Here's how the part is built. I have some questions about the finished solid (model axes, mm). Face numbers are marked on the shaded views. A direction names the side the tool comes from. Round coordinates to 2 decimals unless told otherwise and drop trailing zeros. Order: outer loops, then holes, each group sorted by start corner. A loop starts at its lowest first (then second) coordinate and runs counter-clockwise, first axis right, second up. Notation, with made-up numbers: M 14,-5.75 L 33,-5.75 A12 ccw 33,9.25 Z; hole C -38,82 d3. An arc over 180 degrees is marked long. Use one line per item in the form item = value. Start each with the question number.
```python
from build123d import *

# Parameters (mm, degrees)
SKETCH1_R           = 1.5
SKETCH1_W           = 3
SKETCH1_H           = 3
BOSS_EXTRUDE1_DEPTH = 3
FILLET1_R           = 4


with BuildPart() as part:
    # Sketch1 → Boss-Extrude1 (new body)
    # profile 1 of 3: a face of its own
    with BuildSketch(Plane(origin=(0, 0, 0), x_dir=(1, 0, 0), z_dir=(0, 1, 0))):
        Polygon((14.5, 10), (-1.5, 10), (-1.5, 0), (-8.5, 0), (-11.5, 0), (-14.5, 0), (-14.5, -10), (-11.5, -10), (-8.5, -10), (14.5, -10), align=None)
        with Locations(Location((6.5, 5.75, 0), (0, 0, 270))):
            Circle(SKETCH1_R, mode=Mode.SUBTRACT)
    # profile 2 of 3: a face of its own
    with BuildSketch(Plane(origin=(0, 0, 0), x_dir=(1, 0, 0), z_dir=(0, 1, 0))):
        with Locations((-10, -11.5)):
            Rectangle(SKETCH1_W, SKETCH1_H)
    # profile 3 of 3: a face of its own
    with BuildSketch(Plane(origin=(0, 0, 0), x_dir=(1, 0, 0), z_dir=(0, 1, 0))):
        with Locations((-10, 1.5)):
            Rectangle(SKETCH1_W, SKETCH1_H)
    extrude(amount=BOSS_EXTRUDE1_DEPTH)

    # Fillet1
    # the kernel refuses this fillet: 4 mm, written as the material it adds along each edge
    with BuildSketch(Plane(origin=(-8.5, 0, 0), x_dir=(1, 0, 0), z_dir=(0, 1, 0))) as fillet1_piece_1:
        with BuildLine():
            CenterArc((3.872983346, 4), FILLET1_R, 194.477512186, 75.522487814)
            Line((0, 3), (0, 0))
            Line((0, 0), (3.872983346, 0))
        make_face()
    extrude(amount=3)
    with BuildSketch(Plane(origin=(-8.5, 0, 10), x_dir=(1, 0, 0), z_dir=(0, 1, 0))) as fillet1_piece_2:
        with BuildLine():
            CenterArc((3.872983346, -4), FILLET1_R, 90, 75.522487814)
            Line((0, -3), (0, 0))
            Line((0, 0), (3.872983346, 0))
        make_face()
    extrude(amount=3)
    with BuildSketch(Plane(origin=(-1.5, 0, 0), x_dir=(0, 0, -1), z_dir=(0, 1, 0))) as fillet1_piece_3:
        with BuildLine():
            CenterArc((FILLET1_R, FILLET1_R), FILLET1_R, 180, 90)
            Line((0, FILLET1_R), (0, 0))
            Line((0, 0), (FILLET1_R, 0))
        make_face()
    extrude(amount=3)
    # the kernel refuses this fillet: 4 mm, written as the material it takes off along each edge
    with BuildSketch(Plane(origin=(14.5, -10, 10), x_dir=(0, 0, -1), z_dir=(0, 1, 0)), Plane(origin=(14.5, -10, -10), x_dir=(-1, 0, 0), z_dir=(0, 1, 0))) as fillet1_2_piece_1:
        with BuildLine():
            CenterArc((FILLET1_R, FILLET1_R), FILLET1_R, 180, 90)
            Line((0, FILLET1_R), (0, 0))
            Line((0, 0), (FILLET1_R, 0))
        make_face()
    extrude(amount=23, mode=Mode.SUBTRACT)
    with BuildSketch(Plane(origin=(-1.5, -10, -10), x_dir=(1, 0, 0), z_dir=(0, 1, 0))) as fillet1_2_piece_2:
        with BuildLine():
            CenterArc((FILLET1_R, -FILLET1_R), FILLET1_R, 90, 90)
            Line((0, -FILLET1_R), (0, 0))
            Line((0, 0), (FILLET1_R, 0))
        make_face()
    extrude(amount=23, mode=Mode.SUBTRACT)


solid = part.part
```
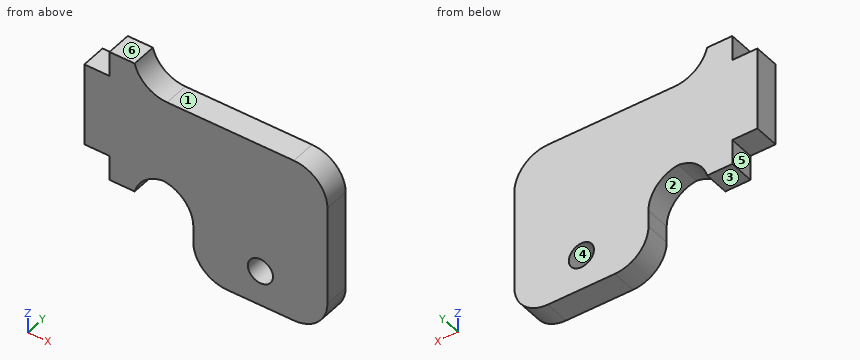
1) If I drill on line 1 (X direction, y = 2.15, z = -5.75); line 2 (X direction, y = 1.75, z = 6.25); line 3 (Z direction, x = 9.25, y = 2.8), over which ranges is the centre line in solid material (lowest first)?
2) On a 3-axis mill with a long thin cutter (end or side, diameter ignored), from which of +Z, -Z, +X, -X, +Y, -Y can I reach the whole of each face in a straight line? I mean the marked faces 1, 2 and 3. Say none if no direction works.
3) If we section it at D-D on x = -9: Write out the boundary of the cut face in (y, z).
4) If we mould it in two halves opening along Z, with no side actions, what happens to the marked faces 4, 5 and 6? For each: +Z half, -Z half, draft (parallel to the pull), parting line (faces both ways), or undercut.
5) If we section it at A-A on x = 6.5: Write out the boundary of the cut face in (y, z).
6) If we section it at B-B on y = 1.4: Write out the boundary of the cut face in (x, z), then the cut area to 3 significant figures.
7) If we section it at C-C on z = -5.25: Write out the boundary of the cut face in (x, y), then the cut area to 3 significant figures.
8) Will these pins go through, and if not, where does the flat tip stop? pin 1 Ø0.9 at (y, z) = (2, -1.5) entering from -X; pin 2 Ø0.9 at (x, y) = (0.5, 1.5) entering from +Z; pin 3 Ø1.5 at (x, y) = (-13, 2) entering from -Z; pin 4 Ø5 at (x, z) = (6.5, -5.75) entering from +Y.
Completed:
q1.line_1 = -1.5 to 5, 8 to 14.5
q1.line_2 = -14.5 to 14.49
q1.line_3 = -10 to 10
q2.face_1 = +Z, +X, +Y, -Y
q2.face_2 = -Z, +Y, -Y
q2.face_3 = -Z, -X, +Y, -Y
q3.outline = M 0,-3 L 3,-3 L 3,13 L 0,13 Z
q4.face_4 = undercut
q4.face_5 = draft
q4.face_6 = +Z half
q5.outline = M 0,-10 L 3,-10 L 3,-7.25 L 0,-7.25 Z; M 0,-4.25 L 3,-4.25 L 3,10 L 0,10 Z
q6.outline = M -14.5,0 L -11.5,0 L -11.5,-3 L -8.5,-3 A4 cw -5.06,-0.02 A4 cw -1.5,-4 L -1.5,-6 A4 ccw 2.5,-10 L 10.5,-10 A4 ccw 14.5,-6 L 14.5,6 A4 ccw 10.5,10 L -4.63,10 A4 cw -8.5,13 L -11.5,13 L -11.5,10 L -14.5,10 Z; hole C 6.5,-5.75 d3
q6.area = 460 mm²
q7.outline = M -1.5,0 L 5.09,0 L 5.09,3 L -1.5,3 Z; M 7.91,0 L 14.5,0 L 14.5,3 L 7.91,3 Z
q7.area = 39.5 mm²
q8.pin_1 = -11.5
q8.pin_2 = 10
q8.pin_3 = 0
q8.pin_4 = 3
